```python
from build123d import *

# Parameters (mm, degrees)
BOSS_EXTRUDE1_DEPTH             = 12.7
BOSS_EXTRUDE4_REACH             = 14.7
BOSS_EXTRUDE4_DIRECTION_2_REACH = 14.7
SKETCH6_W                       = 16.51
SKETCH6_H                       = 15.748
CUT_EXTRUDE2_DEPTH              = 63.23
SKETCH11_W                      = 21.59
SKETCH11_H                      = 7.62
CUT_EXTRUDE3_DEPTH              = 3.81
SKETCH15_R                      = 3.2385
CUT_EXTRUDE4_DEPTH              = 25.4
SKETCH16_W                      = 16.51
SKETCH16_H                      = 12.7
CUT_EXTRUDE5_DEPTH              = 36.83
BOSS_EXTRUDE5_DEPTH             = 5.08
SKETCH18_W                      = 6.35
SKETCH18_H                      = 21.59
BOSS_EXTRUDE6_DEPTH             = 16.51
SKETCH22_W                      = 3.81
SKETCH22_H                      = 3.81
CUT_EXTRUDE6_DEPTH              = 25.4
SKETCH23_W                      = 2.54
SKETCH23_H                      = 4.572
CUT_EXTRUDE7_DEPTH              = 26.4


with BuildPart() as part:
    # Sketch1 → Boss-Extrude1 (new body, symmetric)
    with BuildSketch(Plane.XY):
        with BuildLine():
            Line((-20.32, 16.002), (-20.32, -38.1))
            Line((-20.32, -38.1), (20.32, -38.1))
            Line((20.32, -38.1), (20.32, 16.002))
            Line((20.32, 16.002), (2.794, 16.002))
            Line((2.794, 16.002), (2.794, 28.1305))
            Line((2.794, 28.1305), (6.477, 28.1305))
            ThreePointArc((6.477, 28.1305), (6.946330803, 28.444096816), (6.836210245, 28.997710245))
            Line((6.836210245, 28.997710245), (3.706459265, 32.127461224))
            ThreePointArc((3.706459265, 32.127461224), (2.882423959, 32.678064013), (1.910408041, 32.87141))
            Line((1.910408041, 32.87141), (-1.910408041, 32.87141))
            ThreePointArc((-1.910408041, 32.87141), (-2.882423959, 32.678064013), (-3.706459265, 32.127461224))
            Line((-3.706459265, 32.127461224), (-6.836210245, 28.997710245))
            ThreePointArc((-6.836210245, 28.997710245), (-6.946330803, 28.444096816), (-6.477, 28.1305))
            Line((-6.477, 28.1305), (-2.794, 28.1305))
            Line((-2.794, 28.1305), (-2.794, 16.002))
            Line((-2.794, 16.002), (-20.32, 16.002))
        make_face()
        Polygon((-4.106115114, 7.112), (-8.212230229, 0), (-4.106115114, -7.112), (4.106115114, -7.112), (8.212230229, 0), (4.106115114, 7.112), align=None, mode=Mode.SUBTRACT)
    extrude(amount=BOSS_EXTRUDE1_DEPTH, both=True)

    # Boss-Extrude4: up to this face of the body (flat: up to its plane)
    boss_extrude4_end = Plane(part.part.faces().sort_by_distance((0, -9.949298675, 12.7))[0])
    # Sketch10 → Boss-Extrude4 (add, up to the picked face)
    with BuildSketch(Plane.XY, mode=Mode.PRIVATE) as boss_extrude4_sk1:
        Polygon((-20.32, -38.1), (-20.32, -46.99), (-41.91, -46.99), (-41.91, -50.8), (-16.51, -50.8), (-16.51, -38.1), align=None)
    boss_extrude4_tool1 = split(extrude(boss_extrude4_sk1.sketch, amount=BOSS_EXTRUDE4_REACH, mode=Mode.PRIVATE), bisect_by=boss_extrude4_end, keep=Keep.BOTH, mode=Mode.PRIVATE)
    add(boss_extrude4_tool1.solids().sort_by_distance((-26.411296, -47.248704, 0))[0])

    # Boss-Extrude4 direction 2: up to this face of the body (flat: up to its plane)
    boss_extrude4_direction_2_end = Plane(part.part.faces().sort_by_distance((0, -9.949298675, -12.7))[0])
    # Sketch10 → Boss-Extrude4 direction 2 (add, up to the picked face)
    with BuildSketch(Plane.XY, mode=Mode.PRIVATE) as boss_extrude4_direction_2_sk1:
        Polygon((-20.32, -38.1), (-20.32, -46.99), (-41.91, -46.99), (-41.91, -50.8), (-16.51, -50.8), (-16.51, -38.1), align=None)
    boss_extrude4_direction_2_tool1 = split(extrude(boss_extrude4_direction_2_sk1.sketch, amount=-BOSS_EXTRUDE4_DIRECTION_2_REACH, mode=Mode.PRIVATE), bisect_by=boss_extrude4_direction_2_end, keep=Keep.BOTH, mode=Mode.PRIVATE)
    add(boss_extrude4_direction_2_tool1.solids().sort_by_distance((-26.411296, -47.248704, 0))[0])

    # Sketch6 → Cut-Extrude2 (cut, through all)
    with BuildSketch(Plane(origin=(20.32, 0, 0), x_dir=(0, 0, -1), z_dir=(1, 0, 0))):
        with Locations((0, -17.526)):
            Rectangle(SKETCH6_W, SKETCH6_H)
    extrude(amount=-CUT_EXTRUDE2_DEPTH, mode=Mode.SUBTRACT)

    # Sketch11 → Cut-Extrude3 (cut)
    with BuildSketch(Plane(origin=(0, -46.99, 0), x_dir=(1, 0, 0), z_dir=(0, 1, 0))):
        with Locations((-31.115, 0)):
            Rectangle(SKETCH11_W, SKETCH11_H)
    extrude(amount=-CUT_EXTRUDE3_DEPTH, mode=Mode.SUBTRACT)

    # Sketch15 → Cut-Extrude4 (cut)
    with BuildSketch(Plane.XY.offset(12.7)):
        with Locations((0, -19.05)):
            Circle(SKETCH15_R)
    extrude(amount=-CUT_EXTRUDE4_DEPTH, mode=Mode.SUBTRACT)

    # Sketch16 → Cut-Extrude5 (cut)
    with BuildSketch(Plane(origin=(20.32, 0, 0), x_dir=(0, 0, -1), z_dir=(1, 0, 0))):
        with Locations((0, -31.75)):
            Rectangle(SKETCH16_W, SKETCH16_H)
    extrude(amount=-CUT_EXTRUDE5_DEPTH, mode=Mode.SUBTRACT)

    # Sketch17 → Boss-Extrude5 (add)
    with BuildSketch(Plane.ZY.offset(20.32)):
        Polygon((12.7, -25.4), (12.7, -46.99), (3.81, -46.99), (3.81, -50.8), (-3.81, -50.8), (-3.81, -46.99), (-12.7, -46.99), (-12.7, -25.4), align=None)
    extrude(amount=BOSS_EXTRUDE5_DEPTH)

    # Sketch18 → Boss-Extrude6 (add)
    with BuildSketch(Plane.ZY.offset(25.4)):
        with Locations((-9.525, -36.195)):
            Rectangle(SKETCH18_W, SKETCH18_H)
        with Locations((9.525, -36.195)):
            Rectangle(SKETCH18_W, SKETCH18_H)
    extrude(amount=BOSS_EXTRUDE6_DEPTH)

    # Sketch22 → Cut-Extrude6 (cut)
    with BuildSketch(Plane.XY.offset(12.7)):
        with Locations((-18.415, -48.895)):
            Rectangle(SKETCH22_W, SKETCH22_H)
    extrude(amount=-CUT_EXTRUDE6_DEPTH, mode=Mode.SUBTRACT)

    # Sketch23 → Cut-Extrude7 (cut, through all)
    with BuildSketch(Plane.XY.offset(12.7)):
        with Locations((-38.608, -31.203491357)):
            Rectangle(SKETCH23_W, SKETCH23_H)
        with Locations((-38.608, -41.363491357)):
            Rectangle(SKETCH23_W, SKETCH23_H)
    extrude(amount=-CUT_EXTRUDE7_DEPTH, mode=Mode.SUBTRACT)


solid = part.part
```
The model under review builds one solid part; all positions refer to its coordinate system, in mm. A direction names the side the tool comes from. Coordinates: 2 decimals unless noted, no trailing zeros. Write each loop counter-clockwise with the first axis right and the second up, starting at its lowest first coordinate (ties: lowest second). Pieces come first, ordered by that corner, then holes.
1) To check wall thickness, follow probe 1 along Y at (x, z) = (0, 11.6); probe 2 along Z at (x, y) = (1.5, -13) (3 decimals); probe 3 along Y at (x, z) = (-1.5, -10.5). State the ranges of each line that lie inside material, in increasing order.
2) We need section D-D on x = -17.5. State the section outline as (y, z) points (3 decimals).
3) The part is to be moulded in two halves that separate along Z. For faces 4 (the face through (-34, -49, -3.81)), 5 (the face through (-39.878, -41, 10)), say which applies: pulls with the +Z half, pulls with the -Z half, needs draft (parallel to the pull), parting line crosses it, or undercut.
4) Clearance check with flat-ended pins moving along their axes: pin 1 Ø3.5 at (x, z) = (10.5, 9.5) entering from -Y; pin 2 Ø0.8 at (x, z) = (-38, 10.5) entering from +Y; pin 3 Ø2 at (x, z) = (-37.5, 4.5) entering from +Y; pin 4 Ø4 at (y, z) = (-22.5, -5) entering from -X. State where each tip first meets the part, or that it passes through.
5) We need section C-C on y = -19.05. State the section outline as (x, z) points (1 decimal).
6) We need section B-B on z = 1.5. State the section outline as (x, y) points, then the cut area to 3 significant figures.
7) We need section A-A on x = 0. State the section outline as (y, z) points (1 decimal), then the cut area to 3 significant figures.
8) Machinability: for faces 1 (the face through (-5, 28.13, 0)), 2 (the face through (12, 16.002, 0)), 3 (the face through (-39.878, -31, -9)), which of the approach directions +Z, -Z, +X, -X, +Y, -Y give a long, thin tool a straight path to every point of the face, cutting with its end or side? Answer none if there is none.
Answer list:
1. probe 1: y = -38.1 to -22.29, -15.81 to -7.11, 7.11 to 32.87
1. probe 2: z = -12.7 to -8.255, 8.255 to 12.7
1. probe 3: y = -38.1 to -21.92, -16.18 to -7.11, 7.11 to 32.87
2. outline: (-46.99, -12.7) - (16.002, -12.7) - (16.002, 12.7) - (-46.99, 12.7) - close; hole (-25.4, -8.255) - (-9.652, -8.255) - (-9.652, 8.255) - (-25.4, 8.255) - close
3. face 4: undercut
3. face 5: needs draft
4. pin 1: stops at y = -38.1
4. pin 2: stops at y = -25.4
4. pin 3: stops at y = -46.99
4. pin 4: passes through
5. outline: (-20.3, -12.7) - (-3.2, -12.7) - (-3.2, -8.3) - (-20.3, -8.3) - close; (-20.3, 8.3) - (-3.2, 8.3) - (-3.2, 12.7) - (-20.3, 12.7) - close; (3.2, -12.7) - (20.3, -12.7) - (20.3, -8.3) - (3.2, -8.3) - close; (3.2, 8.3) - (20.3, 8.3) - (20.3, 12.7) - (3.2, 12.7) - close
6. outline: (-25.4, -50.8) - (-20.32, -50.8) - (-20.32, -46.99) - (-16.51, -46.99) - (-16.51, -25.4) - (-25.4, -25.4) - close; (-20.32, -9.65) - (20.32, -9.65) - (20.32, 16) - (2.79, 16) - (2.79, 28.13) - (6.48, 28.13) arc R0.51 ccw to (6.84, 29) - (3.71, 32.13) arc R2.54 ccw to (1.91, 32.87) - (-1.91, 32.87) arc R2.54 ccw to (-3.71, 32.13) - (-6.84, 29) arc R0.51 ccw to (-6.48, 28.13) - (-2.79, 28.13) - (-2.79, 16) - (-20.32, 16) - close; hole (-8.21, 0) - (-4.11, -7.11) - (4.11, -7.11) - (8.21, 0) - (4.11, 7.11) - (-4.11, 7.11) - close
6. area: 1,200 mm2
7. outline: (-38.1, -12.7) - (-22.3, -12.7) - (-22.3, -8.3) - (-38.1, -8.3) - close; (-38.1, 8.3) - (-22.3, 8.3) - (-22.3, 12.7) - (-38.1, 12.7) - close; (-15.8, -12.7) - (-7.1, -12.7) - (-7.1, 12.7) - (-15.8, 12.7) - (-15.8, 8.3) - (-9.7, 8.3) - (-9.7, -8.3) - (-15.8, -8.3) - close; (7.1, -12.7) - (32.9, -12.7) - (32.9, 12.7) - (7.1, 12.7) - close
7. area: 914 mm2
8. face 1: +Z, -Z, -X
8. face 2: +Z, -Z, +X
8. face 3: +Z, -Z
